Part model, mm, in its own coordinate system. A direction names the side the tool comes from. Give positions to 0.01 mm unless a question says otherwise; leave off trailing zeros. Order: outer loops, then holes, each group sorted by start corner. A loop starts at its lowest first (then second) coordinate and runs counter-clockwise, first axis right, second up. Notation, with made-up numbers: M -16,-30 L -6,-30 A27 cw -6,-14 Z; hole C 63,-26 d6. An arc over 180 degrees is marked long. Return JSON: item names as keys, results as strings.
from build123d import *

# Parameters (mm, degrees)
SKETCH1_W           = 319
SKETCH1_H           = 530
BOSS_EXTRUDE1_DEPTH = 265
SKETCH2_W           = 111.097054908
SKETCH2_H           = 215.10280844
BOSS_EXTRUDE2_DEPTH = 120
SKETCH3_R           = 24
BOSS_EXTRUDE3_DEPTH = 110
SKETCH4_W           = 7
SKETCH4_H           = 14
BOSS_EXTRUDE4_DEPTH = 90
FILLET1_R           = 10


with BuildPart() as part:
    # Sketch1 → Boss-Extrude1 (new body)
    with BuildSketch(Plane.XY):
        Rectangle(SKETCH1_W, SKETCH1_H)
    extrude(amount=BOSS_EXTRUDE1_DEPTH)

    # Sketch2 → Boss-Extrude2 (add)
    with BuildSketch(Plane.XY.offset(265)):
        with Locations((0, -134.143784384)):
            Rectangle(SKETCH2_W, SKETCH2_H)
    extrude(amount=BOSS_EXTRUDE2_DEPTH)

    # Sketch3 → Boss-Extrude3 (add)
    with BuildSketch(Plane(origin=(0, 265, 0), x_dir=(1, 0, 0), z_dir=(0, 1, 0))):
        with Locations((-0.5, -160)):
            Circle(SKETCH3_R)
    extrude(amount=BOSS_EXTRUDE3_DEPTH)

    # Sketch4 → Boss-Extrude4 (add)
    with BuildSketch(Plane(origin=(0, 375, 0), x_dir=(1, 0, 0), z_dir=(0, 1, 0))):
        with Locations((-0.5, -184)):
            Rectangle(SKETCH4_W, SKETCH4_H)
    extrude(amount=-BOSS_EXTRUDE4_DEPTH)

    # Fillet1
    fillet1_edges = [part.edges().sort_by_distance(p)[0] for p in [
        (-159.5, 0, 265),
        (0, -265, 265),
        (55.548527454, -134.143784384, 265),
        (55.548527454, -241.695188604, 325),
        (0, -26.592380164, 265),
        (55.548527454, -26.592380164, 325),
        (-55.548527454, -134.143784384, 265),
        (-55.548527454, -26.592380164, 325),
        (0, -241.695188604, 265),
        (-55.548527454, -241.695188604, 325),
        (55.548527454, -134.143784384, 385),
        (0, -26.592380164, 385),
        (-55.548527454, -134.143784384, 385),
        (0, -241.695188604, 385),
        (-24.5, 265, 160),
        (159.5, 0, 265),
        (0, -265, 0),
        (-159.5, 0, 0),
        (0, 265, 0),
        (159.5, 0, 0),
        (0, 265, 265),
        (159.5, -265, 132.5),
        (-159.5, -265, 132.5),
        (-159.5, 265, 132.5),
        (159.5, 265, 132.5),
    ]]
    fillet(fillet1_edges, radius=FILLET1_R)


solid = part.part
Q1. Band-saw the part on C-C (z = 160). Give the cut face in (x, y).
Established:
{"outline": "M -159.5,-255 A10 ccw -149.5,-265 L 149.5,-265 A10 ccw 159.5,-255 L 159.5,255 A10 ccw 149.5,265 L 33.5,265 A10 cw 23.5,275 L 23.5,375 L -24.5,375 L -24.5,275 A10 cw -34.5,265 L -149.5,265 A10 ccw -159.5,255 Z"}
Q2. 3-axis set-ups, long thin cutter, end or side, ignore diameter. For faces 1 (the flat face through (55.549, -136, 324)), 2 (the flat face through (-55.549, -136, 324)), 3 (the flat face through (-1, -241.695, 324)): which of +Z, -Z, +X, -X, +Y, -Y reach the whole face in a straight line?
Established:
{"face 1": "+Z, +X, +Y, -Y", "face 2": "+Z, -X, +Y, -Y", "face 3": "+Z, +X, -X, -Y"}
Q3. Probe line 1 along Z through (x, y) = (-67, 77.5); line 2 along X through (y, z) = (-126, 313.5); line 3 along Y through (x, z) = (-33, 44). List the from-to ranges inside material, lowest first.
Established:
{"line 1": "z = 0 to 265", "line 2": "x = -55.55 to 55.55", "line 3": "y = -265 to 265"}
Q4. Band-saw the part on B-B (z = 292). Give the cut face in (x, y), then the cut area to 3 significant figures.
Established:
{"outline": "M -55.55,-231.7 A10 ccw -45.55,-241.7 L 45.55,-241.7 A10 ccw 55.55,-231.7 L 55.55,-36.59 A10 ccw 45.55,-26.59 L -45.55,-26.59 A10 ccw -55.55,-36.59 Z", "area": "23,800 mm²"}
Q5. Pin check, flat tips, straight feed: pin 1 (1.5 mm diameter, centred on x = 52.5, z = 285.5, fed in from -Y); pin 2 (7.5 mm diameter, centred on x = -0.5, y = 347.5, fed in from +Z); pin 3 (3.5 mm diameter, centred on y = 332.5, z = 189, fed in from +X). Stop position of each tip, or through.
Established:
{"pin 1": "stops at y = -239.54", "pin 2": "stops at z = 191", "pin 3": "stops at x = 3"}
Q6. Band-saw the part on A-A (y = 81). Give the cut face in (x, z), then the cut area to 3 significant figures.
Established:
{"outline": "M -159.5,10 A10 ccw -149.5,0 L 149.5,0 A10 ccw 159.5,10 L 159.5,255 A10 ccw 149.5,265 L -149.5,265 A10 ccw -159.5,255 Z", "area": "84,400 mm²"}
Q7. Band-saw the part on D-D (y = 319.5). Give the cut face in (x, z).
Established:
{"outline": "M -4,183.74 A24 ccw long 3,183.74 L 3,191 L -4,191 Z"}
